```python
from build123d import *

# Parameters (mm, degrees)
ESTRUSIONE_ESTRUSIONE1_DEPTH = 16
RACCORDO1_R                  = 10
RACCORDO2_R                  = 20
SCHIZZO3_R                   = 1.5
TAGLIO_ESTRUSIONE1_DEPTH     = 16
SCHIZZO4_R                   = 2
TAGLIO_ESTRUSIONE2_DEPTH     = 1


with BuildPart() as part:
    # Schizzo1 → Estrusione-Estrusione1 (new body)
    with BuildSketch(Plane.XY):
        with BuildLine():
            Line((3.5, 0), (43, 0))
            Line((43, 0), (43, 1))
            Line((43, 1), (5.949489743, 1))
            ThreePointArc((5.949489743, 1), (6.17260394, 1.240091112), (6.372281323, 1.5))
            Line((6.372281323, 1.5), (34.226351822, 1.5))
            Line((34.226351822, 1.5), (43, 3.047030893))
            Line((43, 3.047030893), (42.826351822, 4.031838646))
            Line((42.826351822, 4.031838646), (34.226351822, 2.515426612))
            Line((34.226351822, 2.515426612), (4.009636789, 6.962696975))
            ThreePointArc((4.009636789, 6.962696975), (0.009338214, 3.755500085), (3.5, 0))
        make_face()
    extrude(amount=ESTRUSIONE_ESTRUSIONE1_DEPTH)

    # Raccordo1
    raccordo1_edges = [part.edges().sort_by_distance(p)[0] for p in [
        (34.226351822, 2.515426612, 8),
    ]]
    fillet(raccordo1_edges, radius=RACCORDO1_R)

    # Raccordo2
    raccordo2_edges = [part.edges().sort_by_distance(p)[0] for p in [
        (34.226351822, 1.5, 8),
    ]]
    fillet(raccordo2_edges, radius=RACCORDO2_R)

    # Schizzo3 → Taglio-Estrusione1 (cut)
    with BuildSketch(Plane.XY.offset(16)):
        with Locations((10, 3.5)):
            Circle(SCHIZZO3_R)
    extrude(amount=-TAGLIO_ESTRUSIONE1_DEPTH, mode=Mode.SUBTRACT)

    # Schizzo4 → Taglio-Estrusione2 (cut)
    with BuildSketch(Plane.XZ):
        with Locations((39, 8)):
            Circle(SCHIZZO4_R)
        with Locations((16, 8)):
            Circle(SCHIZZO4_R)
    extrude(amount=-TAGLIO_ESTRUSIONE2_DEPTH, mode=Mode.SUBTRACT)


solid = part.part
```
The model under review builds one solid part; all positions refer to its coordinate system, in mm. A direction names the side the tool comes from. Give positions to 0.01 mm unless a question says otherwise; leave off trailing zeros. Write each loop counter-clockwise with the first axis right and the second up, starting at its lowest first coordinate (ties: lowest second). Pieces come first, ordered by that corner, then holes.
(1) To check wall thickness, follow L1, parallel to Z at x = 16, y = 0.5; L2, parallel to Y at x = 10.5, z = 15; L3, parallel to Y at x = 10, z = 11.25. State the ranges of each line that lie inside material, in increasing order.
(2) For P1, Ø3, axis at x = 24, z = 8, coming from the +Y side; P2, Ø6.5, axis at x = 16, z = 8, coming from the -Y side; P3, Ø3.5, axis at x = 39, z = 8, coming from the -Y side; P4, Ø8, axis at x = 17, z = 6, coming from the +Y side, all flat-tipped, find the tip position at first contact; note any pin that passes through.
(3) Consider section D-D, the plane z = 1.25. Give the boundary of the cut face in (x, y), and give its area (3 significant figures).
(4) Consider section B-B, the plane y = 4.5. Give the boundary of the cut face in (x, z).
(5) Tool access review of faces 1 (the flat face through (19, 1.5, 8)), 2 (the flat face through (42.914, 3.533, 7.888)), 3 (the flat face through (39.372, 3.423, 7.888)), 4 (the cylindrical face through (37.526, 0.493, 9.352)), 5 (the flat face through (23, 0, 8)): name each direction out of +Z, -Z, +X, -X, +Y, -Y from which nothing blocks a thin tool from reaching the whole face with its end or side.
(6) The part is to be moulded in two halves that separate along Y. For faces 6 (the cylindrical face through (14.526, 0.493, 9.352)), 7 (the flat face through (39.425, 2.417, 7.888)), 8 (the flat face through (18.518, 4.827, 7.888)), 9 (the cylindrical face through (0.016, 3.836, 7.888)), say which applies: released by +Y, released by -Y, zero draft, split by the parting line, or undercut.
(7) Consider section A-A, the plane z = 8. Give the boundary of the cut face in (x, y), and give its area (3 significant figures).
(8) Consider section C-C, the plane x = 16. Give the boundary of the cut face in (y, z).
Returned:
1. L1: z = 0 to 6, 10 to 16
1. L2: y = 0 to 1, 1.5 to 2.09, 4.91 to 6.01
1. L3: y = 0 to 1, 1.5 to 2, 5 to 6.08
2. P1: stops at y = 4.24
2. P2: stops at y = 0
2. P3: stops at y = 2.03
2. P4: stops at y = 5.64
3. outline: (3.5, 0) - (43, 0) - (43, 1) - (5.95, 1) arc R3.5 ccw to (6.37, 1.5) - (32.48, 1.5) arc R20 ccw to (35.95, 1.8) - (43, 3.05) - (42.83, 4.03) - (35.82, 2.8) arc R10 cw to (32.63, 2.75) - (4.01, 6.96) arc R3.5 ccw (long way) to start; hole circle Ø3 at (10, 3.5)
3. area: 163 mm2
4. outline: (0.15, 0) - (8.88, 0) - (8.88, 16) - (0.15, 16) - close; (11.12, 0) - (20.74, 0) - (20.74, 16) - (11.12, 16) - close
5. face 1: +Z, -Z, +X
5. face 2: +Z, -Z, +X, +Y
5. face 3: +Z, -Z, +Y
5. face 4: -Y
5. face 5: +Z, -Z, +X, -X, -Y
6. face 6: zero draft
6. face 7: undercut
6. face 8: released by +Y
6. face 9: split by the parting line
7. outline: (3.5, 0) - (14, 0) - (14, 1) - (5.95, 1) arc R3.5 ccw to (6.37, 1.5) - (32.48, 1.5) arc R20 ccw to (35.95, 1.8) - (43, 3.05) - (42.83, 4.03) - (35.82, 2.8) arc R10 cw to (32.63, 2.75) - (4.01, 6.96) arc R3.5 ccw (long way) to start; (18, 0) - (37, 0) - (37, 1) - (18, 1) - close; (41, 0) - (43, 0) - (43, 1) - (41, 1) - close; hole circle Ø3 at (10, 3.5)
7. area: 155 mm2
8. outline: (0, 0) - (1, 0) - (1, 6) - (0, 6) - close; (0, 10) - (1, 10) - (1, 16) - (0, 16) - close; (1.5, 0) - (5.2, 0) - (5.2, 16) - (1.5, 16) - close
